```python
from build123d import *

# Parameters (mm, degrees)
SKETCH1_R           = 30
SKETCH1_R_2         = 7
BOSS_EXTRUDE1_DEPTH = 10
FILLET1_R           = 10
FILLET2_R           = 20
CUT_EXTRUDE1_START  = 10
CUT_EXTRUDE1_DEPTH  = 5


with BuildPart() as part:
    # Sketch1 → Boss-Extrude1 (new, symmetric)
    with BuildSketch(Plane(origin=(0, 0, 0), x_dir=(1, 0, 0), z_dir=(0, 1, 0))):
        with BuildLine():
            Line((30.700703589, 22.393454382), (128.610913115, 9.761593104))
            ThreePointArc((128.610913115, 9.761593104), (155, 0), (128.610913115, -9.761593104))
            Line((128.610913115, -9.761593104), (30.700703589, -22.393454382))
            ThreePointArc((30.700703589, -22.393454382), (-38, 0), (30.700703589, 22.393454382))
        make_face()
        with Locations(Location((0, 0, 0), (0, 0, 270))):
            Circle(SKETCH1_R, mode=Mode.SUBTRACT)
        with Locations(Location((140, 0, 0), (0, 0, 270))):
            Circle(SKETCH1_R_2, mode=Mode.SUBTRACT)
    extrude(amount=BOSS_EXTRUDE1_DEPTH, both=True)

    # Fillet1
    fillet1_edges = [part.edges().sort_by_distance(p)[0] for p in [
        (128.610913115, 0, -9.761593104),
        (128.610913115, 0, 9.761593104),
    ]]
    fillet(fillet1_edges, radius=FILLET1_R)

    # Fillet2
    fillet2_edges = [part.edges().sort_by_distance(p)[0] for p in [
        (30.700703589, 0, -22.393454382),
        (30.700703589, 0, 22.393454382),
    ]]
    fillet(fillet2_edges, radius=FILLET2_R)

    # Sketch2 → Cut-Extrude1 (cut)
    with BuildSketch(Plane(origin=(0, 0, 0), x_dir=(1, 0, 0), z_dir=(0, 1, 0)).offset(CUT_EXTRUDE1_START)):
        with BuildLine():
            Line((42.097828348, -15.377472859), (126.418285087, -4.498890149))
            ThreePointArc((126.418285087, -4.498890149), (130.818347989, 0), (126.418285087, 4.498890149))
            Line((126.418285087, 4.498890149), (42.097828348, 15.377472859))
            ThreePointArc((42.097828348, 15.377472859), (38.350242622, 14.602706981), (36.248141548, 11.404921495))
            ThreePointArc((36.248141548, 11.404921495), (38, 0), (36.248141548, -11.404921495))
            ThreePointArc((36.248141548, -11.404921495), (38.350242622, -14.602706981), (42.097828348, -15.377472859))
        make_face()
    extrude(amount=-CUT_EXTRUDE1_DEPTH, mode=Mode.SUBTRACT)


solid = part.part
```
Design review of the part built by this model. Coordinates are the model's own, in mm. A direction names the side the tool comes from. Coordinates: 2 decimals unless noted, no trailing zeros. Write each loop counter-clockwise with the first axis right and the second up, starting at its lowest first coordinate (ties: lowest second). Pieces come first, ordered by that corner, then holes.
1) Add section A-A (z = 0). Write out the cut boundary in (x, y).
2) Add section B-B (x = 0). Write out the cut boundary in (y, z).
3) Insertion check: pin 1 (8.5 mm diameter, centred on x = 140, z = 0, fed in from +Y) (1 decimal); pin 2 (2 mm diameter, centred on y = 7.5, z = -24, fed in from +X); pin 3 (1.5 mm diameter, centred on x = 52, y = 0, fed in from -Z); pin 4 (3 mm diameter, centred on x = 9.5, y = -4, fed in from +Z). Each pin has a flat end and moves straight along its axis. Give the tip position at first contact, or say it passes through.
4) Machinability: for faces 1 (the flat face through (60, -10, -1)), 2 (the cylindrical face through (130.817, 7.535, 0.098)), 3 (the flat face through (81.74, 0.14, 15.81)), which of the approach directions +Z, -Z, +X, -X, +Y, -Y give a long, thin tool a straight path to every point of the face, cutting with its end or side? Answer none if there is none.
5) Add section C-C (y = 7). Write out the cut boundary in (x, z), plus the area to 3 significant figures.
6) Mouldability with a two-part tool opening along X and no side actions: class faces 4 (the cylindrical face through (31.912, 0.14, 23.326)), 5 (the flat face through (83.668, 7.535, 10.014)), 6 (the flat face through (80.54, 0.14, -15.963)), 7 (the cylindrical face through (-37.98, 0.14, 1.25)) as +X half, -X half, draft (parallel to the pull), parting line (faces both ways), or undercut.
7) To check wall thickness, follow L1, parallel to X at y = -5.5, z = 0; L2, parallel to X at y = 2.75, z = 7.5; L3, parallel to Z at x = 20, y = -0.25. State the ranges of each line that lie inside material, in increasing order.
8) Add section D-D (y = -6). Write out the cut boundary in (x, z), plus the area to 3 significant figures.
Check result:
1. outline: (-38, -10) - (-30, -10) - (-30, 10) - (-38, 10) - close; (30, -10) - (133, -10) - (133, 10) - (130.82, 10) - (130.82, 5) - (38, 5) - (38, 10) - (30, 10) - close; (147, -10) - (155, -10) - (155, 10) - (147, 10) - close
2. outline: (-10, -38) - (10, -38) - (10, -30) - (-10, -30) - close; (-10, 30) - (10, 30) - (10, 38) - (-10, 38) - close
3. pin 1: passes through
3. pin 2: stops at x = 32.61
3. pin 3: stops at z = -19.74
3. pin 4: stops at z = 37.15
4. face 1: +Z, -Z, +X, -X, -Y
4. face 2: +Y
4. face 3: +Z, +Y, -Y
5. outline: (26.71, -27.03) arc R20 cw to (38.2, -21.43) - (124.08, -10.35) arc R10 cw to (131.22, -12.16) arc R15 ccw (long way) to (131.22, 12.16) arc R10 cw to (124.08, 10.35) - (38.2, 21.43) arc R20 cw to (26.71, 27.03) arc R38 ccw (long way) to start; hole circle Ø60 at (0, 0); hole (36.25, -11.4) arc R5 ccw to (42.1, -15.38) - (126.42, -4.5) arc R4.5 ccw to (126.42, 4.5) - (42.1, 15.38) arc R5 ccw to (36.25, 11.4) arc R38 cw to start; hole circle Ø14 at (140, 0)
5. area: 3,310 mm2
6. face 4: +X half
6. face 5: undercut
6. face 6: undercut
6. face 7: parting line
7. L1: x = -38 to -30, 30 to 133, 147 to 155
7. L2: x = -37.25 to -29.05, 29.05 to 152.99
7. L3: z = -32.31 to -22.36, 22.36 to 32.31
8. outline: (26.71, -27.03) arc R20 cw to (38.2, -21.43) - (124.08, -10.35) arc R10 cw to (131.22, -12.16) arc R15 ccw (long way) to (131.22, 12.16) arc R10 cw to (124.08, 10.35) - (38.2, 21.43) arc R20 cw to (26.71, 27.03) arc R38 ccw (long way) to start; hole circle Ø60 at (0, 0); hole circle Ø14 at (140, 0)
8. area: 5,160 mm2
